from build123d import *

# Parameters (mm, degrees)
EXTRUDE_2_DEPTH     = 3
SKETCH_11_R         = 1.7
CUT_EXTRUDE_2_DEPTH = 82.688432474
SKETCH_13_W         = 35.5
SKETCH_13_H         = 21
CUT_EXTRUDE_3_DEPTH = 0.6
SKETCH_14_W         = 12
SKETCH_14_H         = 8.5
CUT_EXTRUDE_4_DEPTH = 82.668598617
SKETCH_16_R         = 3.1
CUT_EXTRUDE_5_DEPTH = 1.5
SKETCH_17_R         = 3.35
CUT_EXTRUDE_6_DEPTH = 0.5


with BuildPart() as part:
    # 草图8 → 凸台-拉伸2 (new body)
    with BuildSketch(Plane(origin=(0, 0, 0), x_dir=(1, 0, 0), z_dir=(0, 1, 0))):
        with BuildLine():
            Line((-21.65, 30), (66.65, 30))
            ThreePointArc((66.65, 30), (69.018807717, 29.018807717), (70, 26.65))
            Line((70, 26.65), (70, -38.65))
            ThreePointArc((70, -38.65), (69.018807717, -41.018807717), (66.65, -42))
            Line((66.65, -42), (-21.65, -42))
            ThreePointArc((-21.65, -42), (-24.018807717, -41.018807717), (-25, -38.65))
            Line((-25, -38.65), (-25, 26.65))
            ThreePointArc((-25, 26.65), (-24.018807717, 29.018807717), (-21.65, 30))
        make_face()
    extrude(amount=EXTRUDE_2_DEPTH)

    # 草图11 → 切除-拉伸2 (cut, through all)
    with BuildSketch(Plane(origin=(0, 3, 0), x_dir=(1, 0, 0), z_dir=(0, 1, 0))):
        with Locations(Location((-19.5, 23.71, 0), (0, 0, 270))):
            Circle(SKETCH_11_R)
        with Locations(Location((-19.5, -36.29, 0), (0, 0, 270))):
            Circle(SKETCH_11_R)
        with Locations(Location((50.5, 23.71, 0), (0, 0, 270))):
            Circle(SKETCH_11_R)
        with Locations(Location((50.5, -36.29, 0), (0, 0, 270))):
            Circle(SKETCH_11_R)
    extrude(amount=-CUT_EXTRUDE_2_DEPTH, mode=Mode.SUBTRACT)

    # 草图13 → 切除-拉伸3 (cut)
    with BuildSketch(Plane(origin=(0, 3, 0), x_dir=(1, 0, 0), z_dir=(0, 1, 0))):
        with Locations((1.176, -6.295)):
            Rectangle(SKETCH_13_W, SKETCH_13_H)
    extrude(amount=-CUT_EXTRUDE_3_DEPTH, mode=Mode.SUBTRACT)

    # 草图14 → 切除-拉伸4 (cut, through all)
    with BuildSketch(Plane(origin=(0, 2.4, 0), x_dir=(1, 0, 0), z_dir=(0, 1, 0))):
        with Locations((0, -6.29)):
            Rectangle(SKETCH_14_W, SKETCH_14_H)
    extrude(amount=-CUT_EXTRUDE_4_DEPTH, mode=Mode.SUBTRACT)

    # 草图16 → 切除-拉伸5 (cut)
    with BuildSketch(Plane.XZ):
        with Locations(Location((-19.5, 36.29, 0), (0, 0, 270))):
            Circle(SKETCH_16_R)
        with Locations(Location((-19.5, -23.71, 0), (0, 0, 270))):
            Circle(SKETCH_16_R)
        with Locations(Location((50.5, 36.29, 0), (0, 0, 270))):
            Circle(SKETCH_16_R)
        with Locations(Location((50.5, -23.71, 0), (0, 0, 270))):
            Circle(SKETCH_16_R)
    extrude(amount=-CUT_EXTRUDE_5_DEPTH, mode=Mode.SUBTRACT)

    # 草图17 → 切除-拉伸6 (cut)
    with BuildSketch(Plane.XZ):
        with Locations(Location((-19.5, 36.29, 0), (0, 0, 270))):
            Circle(SKETCH_17_R)
        with Locations(Location((-19.5, -23.71, 0), (0, 0, 270))):
            Circle(SKETCH_17_R)
        with Locations(Location((50.5, 36.29, 0), (0, 0, 270))):
            Circle(SKETCH_17_R)
        with Locations(Location((50.5, -23.71, 0), (0, 0, 270))):
            Circle(SKETCH_17_R)
    extrude(amount=-CUT_EXTRUDE_6_DEPTH, mode=Mode.SUBTRACT)


solid = part.part
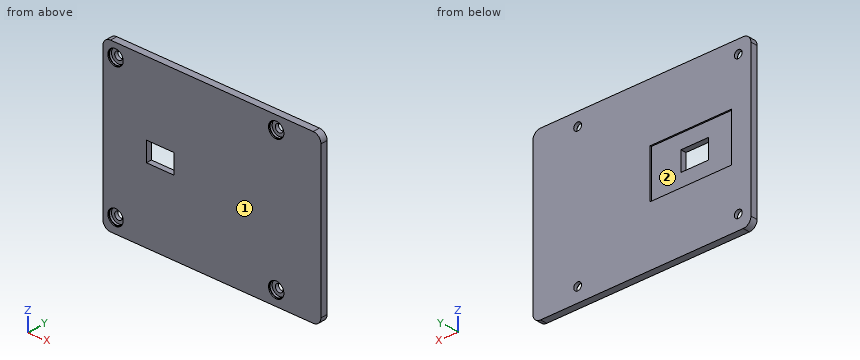
Here's how the part is built. I have some questions about the finished solid (model axes, mm). Face numbers are marked on the shaded views. Coordinates: 2 decimals unless noted, no trailing zeros. Write each loop counter-clockwise with the first axis right and the second up, starting at its lowest first coordinate (ties: lowest second). Pieces come first, ordered by that corner, then holes.
1) I'm going to push flat-ended pins straight in: pin 1 (3 mm diameter, centred on x = -20, z = 35.5, fed in from -Y); pin 2 (6.5 mm diameter, centred on x = -4.5, z = 6.5, fed in from +Y). Where does each tip first touch, or does it pass through?
Filled in:
pin 1: stops at y = 1.5
pin 2: stops at y = 2.4
2) Thinking about a two-plate mould opening in Z: for the marked faces 1 and 2, which applies, +Z half, -Z half, draft (parallel to the pull), parting line (faces both ways), or undercut?
Filled in:
face 1: draft
face 2: undercut
3) If we section it at C-C (x = 50.5): List the corners of the cut face in (y, z) for me, plus the area to 3 significant figures.
Filled in:
outline: (0, -30) - (3, -30) - (3, -25.41) - (1.5, -25.41) - (1.5, -26.81) - (0.5, -26.81) - (0.5, -27.06) - (0, -27.06) - close; (0, -20.36) - (0.5, -20.36) - (0.5, -20.61) - (1.5, -20.61) - (1.5, -22.01) - (3, -22.01) - (3, 34.59) - (1.5, 34.59) - (1.5, 33.19) - (0.5, 33.19) - (0.5, 32.94) - (0, 32.94) - close; (0, 39.64) - (0.5, 39.64) - (0.5, 39.39) - (1.5, 39.39) - (1.5, 37.99) - (3, 37.99) - (3, 42) - (0, 42) - close
area: 187 mm2
4) If I drill on line 1 (X direction, y = 1.95, z = -23.71); line 2 (X direction, y = 0.15, z = 36.29); line 3 (X direction, y = 2.8, z = -4), over which ranges is the centre line in solid material (lowest first)?
Filled in:
line 1: x = -25 to -21.2, -17.8 to 48.8, 52.2 to 70
line 2: x = -25 to -22.85, -16.15 to 47.15, 53.85 to 70
line 3: x = -25 to -16.57, 18.93 to 70
5) If we section it at D-D (z = -2.5): List the corners of the cut face in (x, y) for me.
Filled in:
outline: (-25, 0) - (70, 0) - (70, 3) - (18.93, 3) - (18.93, 2.4) - (-16.57, 2.4) - (-16.57, 3) - (-25, 3) - close
6) If we section it at A-A (z = 36.29): List the corners of the cut face in (x, y) for me, plus the area to 3 significant figures.
Filled in:
outline: (-25, 0) - (-22.85, 0) - (-22.85, 0.5) - (-22.6, 0.5) - (-22.6, 1.5) - (-21.2, 1.5) - (-21.2, 3) - (-25, 3) - close; (-17.8, 1.5) - (-16.4, 1.5) - (-16.4, 0.5) - (-16.15, 0.5) - (-16.15, 0) - (47.15, 0) - (47.15, 0.5) - (47.4, 0.5) - (47.4, 1.5) - (48.8, 1.5) - (48.8, 3) - (-17.8, 3) - close; (52.2, 1.5) - (53.6, 1.5) - (53.6, 0.5) - (53.85, 0.5) - (53.85, 0) - (70, 0) - (70, 3) - (52.2, 3) - close
area: 256 mm2
7) If we section it at B-B (y = 1): List the corners of the cut face in (x, z) for me.
Filled in:
outline: (-25, -26.65) arc R3.35 ccw to (-21.65, -30) - (66.65, -30) arc R3.35 ccw to (70, -26.65) - (70, 38.65) arc R3.35 ccw to (66.65, 42) - (-21.65, 42) arc R3.35 ccw to (-25, 38.65) - close; hole circle Ø6.2 at (-19.5, -23.71); hole circle Ø6.2 at (-19.5, 36.29); hole (-6, 2.04) - (6, 2.04) - (6, 10.54) - (-6, 10.54) - close; hole circle Ø6.2 at (50.5, -23.71); hole circle Ø6.2 at (50.5, 36.29)
